from build123d import *

# Parameters (mm, degrees)
SKETCH2_R           = 2.05
BOSS_EXTRUDE1_DEPTH = 97.028
CUT_EXTRUDE2_DEPTH  = 19.465030121


with BuildPart() as part:
    # Sketch2 → Boss-Extrude1 (new body)
    with BuildSketch(Plane(origin=(0, 0, 0), x_dir=(0, 0, -1), z_dir=(1, 0, 0))):
        with BuildLine():
            Line((-26.512665251, 4.5), (-3, 4.5))
            Line((-3, 4.5), (0, 4.5))
            Line((0, 4.5), (0, 7.5))
            Line((0, 7.5), (0, 35.905))
            ThreePointArc((0, 35.905), (0.352126006, 36.382632999), (0.912533128, 36.187517996))
            Line((0.912533128, 36.187517996), (7.300265025, 26.86014397))
            ThreePointArc((7.300265025, 26.86014397), (7.829571496, 23.444845397), (5.5, 20.891900756))
            Line((5.5, 20.891900756), (5.5, 14.006277796))
            ThreePointArc((5.5, 14.006277796), (6.490325157, 13.388297873), (7.247328797, 12.499709897))
            ThreePointArc((7.247328797, 12.499709897), (7.423857579, 4.201101474), (0.265030121, 0))
            Line((0.265030121, 0), (-22.684455065, 0))
            ThreePointArc((-22.684455065, 0), (-23.989716987, -0.085551386), (-25.272645516, -0.340741737))
            Line((-25.272645516, -0.340741737), (-35.31052949, -3.030384642))
            ThreePointArc((-35.31052949, -3.030384642), (-36.942206253, -2.420445594), (-36.896944076, -0.679082324))
            ThreePointArc((-36.896944076, -0.679082324), (-32.314736873, 3.133398682), (-26.512665251, 4.5))
        make_face()
        with Locations((4, 24.6)):
            Circle(SKETCH2_R, mode=Mode.SUBTRACT)
        with Locations((4, 10.5)):
            Circle(SKETCH2_R, mode=Mode.SUBTRACT)
    extrude(amount=BOSS_EXTRUDE1_DEPTH)

    # Sketch4 → Cut-Extrude2 (cut, through all)
    with BuildSketch(Plane.XY.offset(10)):
        with BuildLine():
            Line((26, 7), (26, 32.405))
            ThreePointArc((26, 32.405), (24.828427125, 35.233427125), (22, 36.405))
            Line((22, 36.405), (75.028, 36.405))
            ThreePointArc((75.028, 36.405), (72.199572875, 35.233427125), (71.028, 32.405))
            Line((71.028, 32.405), (71.028, 7))
            ThreePointArc((71.028, 7), (70.735106781, 6.292893219), (70.028, 6))
            Line((70.028, 6), (66.028, 6))
            ThreePointArc((66.028, 6), (65.320893219, 6.292893219), (65.028, 7))
            Line((65.028, 7), (65.028, 10))
            ThreePointArc((65.028, 10), (63.856427125, 12.828427125), (61.028, 14))
            Line((61.028, 14), (36, 14))
            ThreePointArc((36, 14), (33.171572875, 12.828427125), (32, 10))
            Line((32, 10), (32, 7))
            ThreePointArc((32, 7), (31.707106781, 6.292893219), (31, 6))
            Line((31, 6), (27, 6))
            ThreePointArc((27, 6), (26.292893219, 6.292893219), (26, 7))
        make_face()
    extrude(amount=-CUT_EXTRUDE2_DEPTH, mode=Mode.SUBTRACT)


solid = part.part
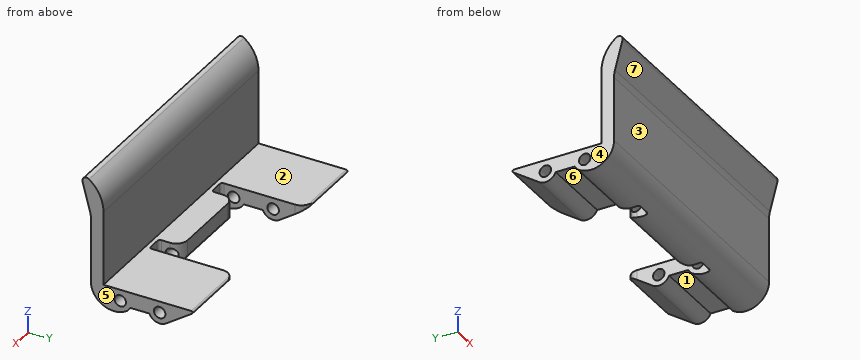
Source: CAD feature listing. Evaluate the final solid. Frame: model axes, mm. Face numbers are marked on the shaded views. A direction names the side the tool comes from. Coordinates: 2 decimals unless noted, no trailing zeros. Loops run counter-clockwise (first coordinate to the right, second up) from the corner with the lowest first, then second, coordinate; pieces in that order, holes last. Notation, with made-up numbers: (-39, 89.25) - (-31, 89.25) arc R7 ccw to (-31, 95.25) - close; hole circle Ø2 at (-3, 37.25). An arc over 180 degrees is marked (long way). Return JSON: item names as keys, results as strings.
Q1. Section D-D, the plane x = 30. Return loops of the section in (y, z).
Results:
{"outline": "(-3.03, 35.31) - (-0.34, 25.27) arc R10 cw to (0, 22.68) - (0, -0.27) arc R8.2 ccw to (6, -8.16) - (6, 0) - (4.5, 0) - (4.5, 26.51) arc R13 ccw to (-0.68, 36.9) arc R1.5 ccw to start"}
Q2. Material intervals for line 1 along X through (y, z) = (7, -4.5); line 2 along Y through (x, z) = (82.5, -3); line 3 along Y through (x, z) = (20, -4), sorted ascending.
Results:
{"line 1": "0 to 26, 32 to 65.03, 71.03 to 97.03", "line 2": "0.47 to 8.71, 12.29 to 22.81, 26.39 to 33.14", "line 3": "0.9 to 8.45, 12.55 to 22.55, 26.65 to 31.68"}
Q3. Section C-C, the plane x = 11. Give the number of separate pieces and of enclosed holes in the cut face, plus the area to 3 significant figures.
Results:
{"separate pieces": "1", "enclosed holes": "2", "area": "366 mm2"}
Q4. Access query for the marked faces 1, 2, 3 and 4. Directions: +Z, -Z, +X, -X, +Y, -Y. A direction counts if a zero-diameter tool reaches every point of the face in a straight line with its end or side. Return the directions, or none.
Results:
{"face 1": "-Z, +X, -X", "face 2": "+Z, +X, -X, +Y", "face 3": "-Z, +X, -X, -Y", "face 4": "+Z, -Z, -X, +Y, -Y"}
Q5. Contact query for flat-ended pins moving along their axis: P1, Ø6, axis at x = 43, z = -2.5, coming from the +Y side; P2, Ø3.5, axis at x = 78, y = 18, coming from the -Z side; P3, Ø5, axis at x = 13, z = 29, coming from the -Y side. Output: stop coordinate, or through.
Results:
{"P1": "y = 14", "P2": "z = -5.5", "P3": "y = -2.01"}
Q6. Section B-B, the plane y = 16. Return loops of the section in (x, z).
Results:
{"outline": "(0, -5.5) - (26, -5.5) - (26, 0) - (0, 0) - close; (71.03, -5.5) - (97.03, -5.5) - (97.03, 0) - (71.03, 0) - close"}
Q7. Mould query, pull axis Y, two halves, no side actions, for the marked faces 5, 6 and 7. Classes: released by +Y, released by -Y, zero draft, split by the parting line, or undercut.
Results:
{"face 5": "zero draft", "face 6": "undercut", "face 7": "released by -Y"}
Q8. Section A-A, the plane y = 24.6. Return loops of the section in (x, z).
Results:
{"outline": "(0, -8) - (26, -8) - (26, -6.05) - (0, -6.05) - close; (0, -1.95) - (26, -1.95) - (26, 0) - (0, 0) - close; (71.03, -8) - (97.03, -8) - (97.03, -6.05) - (71.03, -6.05) - close; (71.03, -1.95) - (97.03, -1.95) - (97.03, 0) - (71.03, 0) - close"}
